Autodesk Inventor part; units mm, degrees
ref_plane "YZ Plane" through (0, 0, 0) normal (1, 0, 0) x (0, 1, 0)
ref_plane "XZ Plane" through (0, 0, 0) normal (0, 1, 0) x (-1, 0, 0)
ref_plane "XY Plane" through (0, 0, 0) normal (0, 0, 1) x (1, 0, 0)
sketch "Sketch1" plane through (0, 0, 0) normal (0, 1, 0) x (-1, 0, 0)
  circle A0 centre (0, 0) radius 30
  line L0 (64.9519, -37.5) -> (0, -75)
  line L1 (0, -75) -> (-64.9519, -37.5)
  line L2 (-64.9519, -37.5) -> (-64.9519, 37.5)
  line L3 (-64.9519, 37.5) -> (0, 75)
  line L4 (0, 75) -> (64.9519, 37.5)
  line L5 (64.9519, 37.5) -> (64.9519, -37.5)
  line L6 (58.5619, 31.7388) -> (52.2358, 31.7388)
  line L7 (52.2358, 31.7388) -> (52.2358, 12.78)
  line L8 (52.2358, 12.78) -> (58.5619, 12.78)
  line L9 (58.5619, 12.78) -> (58.5619, 31.7388)
  line L10 (64.9519, 0) -> (0, 0) construction
  line L11 (58.5619, -31.7388) -> (52.2358, -31.7388)
  line L12 (52.2358, -31.7388) -> (52.2358, -12.78)
  line L13 (52.2358, -12.78) -> (58.5619, -12.78)
  line L14 (58.5619, -12.78) -> (58.5619, -31.7388)
  line L15 (-40.3488, 44.3261) -> (-56.7676, 34.8467)
  line L16 (-56.7676, 34.8467) -> (-53.6045, 29.3681)
  line L17 (-53.6045, 29.3681) -> (-37.1857, 38.8475)
  line L18 (-37.1857, 38.8475) -> (-40.3488, 44.3261)
  line L19 (-15.0501, 51.6275) -> (-18.2131, 57.1061)
  line L20 (-18.2131, 57.1061) -> (-1.7943, 66.5855)
  line L21 (-1.7943, 66.5855) -> (1.3687, 61.1069)
  line L22 (1.3687, 61.1069) -> (-15.0501, 51.6275)
  line L23 (-18.2131, -57.1061) -> (-1.7943, -66.5855)
  line L24 (-1.7943, -66.5855) -> (1.3687, -61.1069)
  line L25 (1.3687, -61.1069) -> (-15.0501, -51.6275)
  line L26 (-15.0501, -51.6275) -> (-18.2131, -57.1061)
  line L27 (-37.1857, -38.8475) -> (-40.3488, -44.3261)
  line L28 (-40.3488, -44.3261) -> (-56.7676, -34.8467)
  line L29 (-56.7676, -34.8467) -> (-53.6045, -29.3681)
  line L30 (-53.6045, -29.3681) -> (-37.1857, -38.8475)
  line L31 (55.3989, -12.78) -> (55.3989, 12.78) construction
  dimension "d0" = 60
  dimension "d3" = 6.3261
  dimension "d4" = 18.9588
  dimension "d5" = 6.39
  dimension "d6" = 12.78
  dimension "d9" = 360
  dimension "d13" = 75
  dimension "d14" = 150
  dimension "LightDiskArm" = 55.3989
  dimension "d16" = 58.5619
  dimension "d17" = 129.9038
extrude "Extrusion1" add sketch "Sketch1" along normal blind 6.39
equation "\"d3\" = 0.99 * WoodThickness"
equation "\"d4\" = 0.25 * DiskGap"
equation "\"d5\" = WoodThickness"
equation "\"d6\" = 2 * WoodThickness"
equation "\"d11\" = WoodThickness"
properties part number "LightDiskBottom" material "MDF Medium Density Fiberboard"
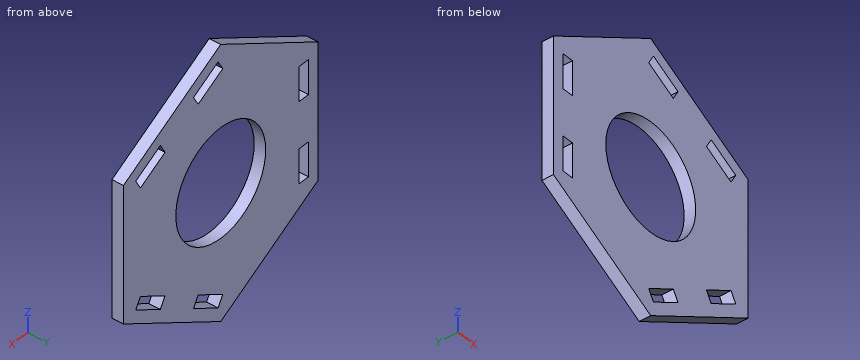
Could you check a few things on this model? Use its own coordinates, in mm. Round coordinates to 2 decimals unless told otherwise and drop trailing zeros. Loops run counter-clockwise (first coordinate to the right, second up) from the corner with the lowest first, then second, coordinate; pieces in that order, holes last.
Q1. I want a section at A-A (z = 0). Write out the boundary of the cut face in (x, y).
Q2. I want a section at C-C (x = -17.5). Write out the boundary of the cut face in (y, z), and give its area (3 significant figures).
Q3. I want a section at B-B (y = 4.5). Give the number of separate pieces and of enclosed holes in the cut face, and give its area (3 significant figures).
Q4. For P1, Ø1.9, axis at x = -54.5, y = 3.5, coming from the -Z side; P2, Ø1.5, axis at x = 51.5, y = 2, coming from the -Z side; P3, Ø3, axis at x = -57, y = 2, coming from the -Z side, each with a flat end and sliding along its axis, tell me the tip position at first contact or that it passes through.
Q5. Please list where these lines run through material, in increasing order: L1, parallel to Z at x = 0, y = 2.25; L2, parallel to X at y = 4.5, z = -38; L3, parallel to Z at x = -12, y = 2.
Answer below:
1. outline: (-64.95, 0) - (-30, 0) - (-30, 6.39) - (-64.95, 6.39) - close; (30, 0) - (64.95, 0) - (64.95, 6.39) - (30, 6.39) - close
2. outline: (0, -64.9) - (6.39, -64.9) - (6.39, -24.37) - (0, -24.37) - close; (0, 24.37) - (6.39, 24.37) - (6.39, 64.9) - (0, 64.9) - close
2. area: 518 mm2
3. separate pieces: 1
3. enclosed holes: 7
3. area: 11,100 mm2
4. P1: stops at z = -44.08
4. P2: stops at z = -45.7
4. P3: stops at z = -42.96
5. L1: z = -75 to -63.48, -60.32 to -30, 30 to 60.32, 63.48 to 75
5. L2: x = -64.09 to 38.65, 51.31 to 64.09
5. L3: z = -68.07 to -27.5, 27.5 to 68.07
